The figure shows three views and two pictorial views of one solid part (mm, origin at its lowest corner). Answer the questions. Give positions to 0.01 mm unless a question says otherwise; leave off trailing zeros. Loops run counter-clockwise (first coordinate to the right, second up) from the corner with the lowest first, then second, coordinate; pieces in that order, holes last.
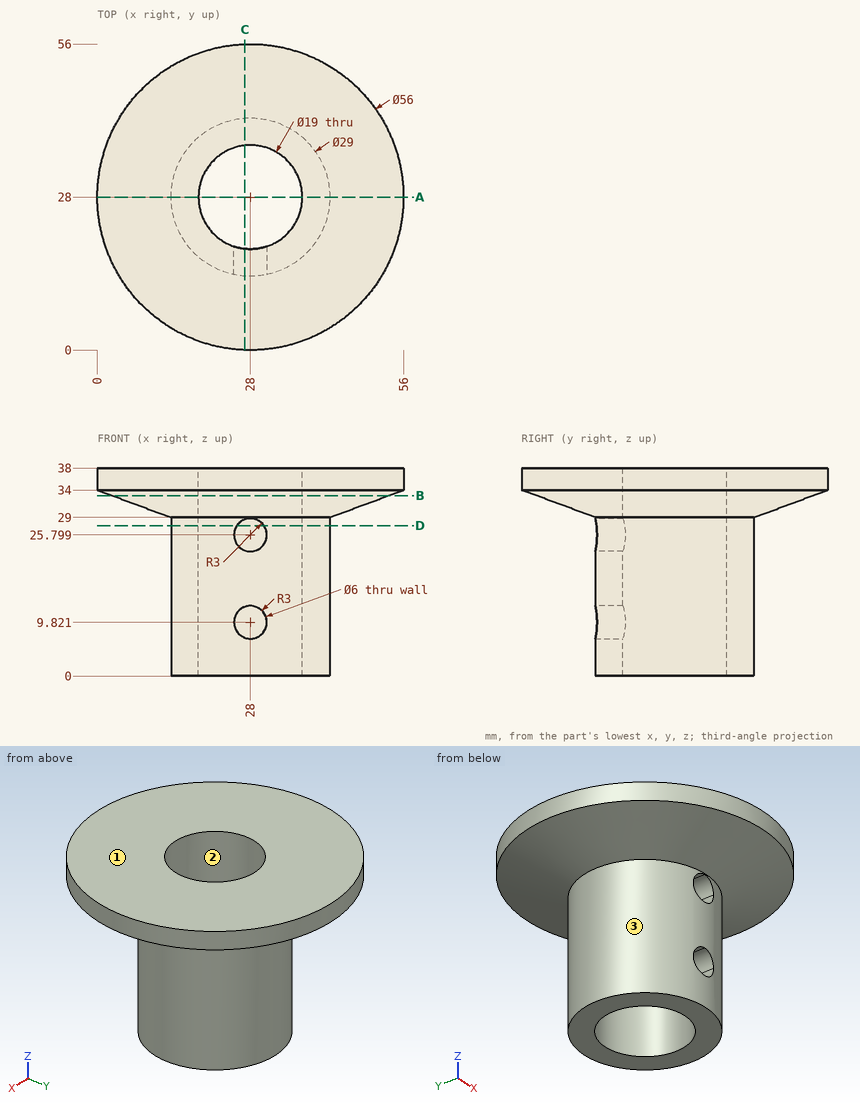
Q1. Consider line 1 along Z through (x, y) = (28, 14.65); line 2 along Y through (x, z) = (27, 36); line 3 along X through (y, z) = (26, 12). Determine where each line is inside the solid, lowest interval first.
Q2. Determine the mould class of the marked faces 1, 2 and 3 for opening direction X: +X half, -X half, draft (parallel to the pull), parting line (faces both ways), or undercut.
Q3. Section D-D on z = 27.5 is taken. Give the vertices of the cut face in (x, y), plus the area to 3 significant figures.
Q4. Given pin 1 (4 mm diameter, centred on x = 37, z = 26, fed in from +Y); pin 2 (10 mm diameter, centred on x = 20, z = 20, fed in from +Y); pin 3 (6 mm diameter, centred on y = 12.5, z = 33, fed in from +X); pin 4 (17 mm diameter, centred on x = 28, y = 28, fed in from +Z), each flat-ended and moving along its own axis, determine where each tip first touches the part or whether it passes through.
Q5. Section B-B on z = 33 is taken. Give the vertices of the cut face in (x, y).
Q6. Section A-A on y = 28 is taken. Give the vertices of the cut face in (x, z).
Q7. Section C-C on x = 27 is taken. State how many separate pieces and enclosed holes the cut face has, plus the area to 3 significant figures.
Check result:
1. line 1: z = 0 to 6.82, 12.82 to 22.8, 28.8 to 38
1. line 2: y = 0.02 to 18.55, 37.45 to 55.98
1. line 3: x = 13.64 to 18.71, 37.29 to 42.36
2. face 1: draft
2. face 2: undercut
2. face 3: parting line
3. outline: (25.53, 13.71) - (25.53, 18.83) arc R9.5 cw (long way) to (30.47, 18.83) - (30.47, 13.71) arc R14.5 ccw (long way) to start
3. area: 352 mm2
4. pin 1: stops at y = 40.7
4. pin 2: stops at y = 42.19
4. pin 3: stops at x = 52.97
4. pin 4: passes through
5. outline: circle Ø50.6 at (28, 28); hole circle Ø19 at (28, 28)
6. outline: (0, 34) - (13.5, 29) - (13.5, 0) - (18.5, 0) - (18.5, 38) - (0, 38) - close; (37.5, 0) - (42.5, 0) - (42.5, 29) - (56, 34) - (56, 38) - (37.5, 38) - close
7. separate pieces: 4
7. enclosed holes: 0
7. area: 500 mm2
